Can you work these out from the model? Positions are in its coordinate system, mm. A direction names the side the tool comes from. Round coordinates to 2 decimals unless told otherwise and drop trailing zeros. Order: outer loops, then holes, each group sorted by start corner. A loop starts at its lowest first (then second) coordinate and runs counter-clockwise, first axis right, second up. Notation, with made-up numbers: M 86,74 L 106,74 A34 ccw 106,104 Z; hole C 21.5,-16.75 d3. An arc over 180 degrees is marked long. Answer as a JSON object with one key per item and string values. Group by question number.
```python
from build123d import *

# Parameters (mm, degrees)
ESQUISSE1_W                  = 62
ESQUISSE1_H                  = 62
BOSS_EXTRU_1_DEPTH           = 68
ESQUISSE2_R                  = 19
BOSS_EXTRU_2_DEPTH           = 4
ESQUISSE3_R                  = 8
BOSS_EXTRU_3_DEPTH           = 5
ENL_V_MAT_EXTRU_1_DEPTH      = 111.959452053
ENL_V_MAT_EXTRU_1_DEPTH_BACK = 111.959452053
ESQUISSE4_R                  = 3.6
CHANFREIN1_SIZE              = 3
ESQUISSE5_W                  = 20
ESQUISSE5_H                  = 9.5
BOSS_EXTRU_4_DEPTH           = 68
ESQUISSE6_R                  = 4.7625
ENL_V_MAT_EXTRU_2_DEPTH      = 5
ESQUISSE7_R                  = 5
ENL_V_MAT_EXTRU_3_DEPTH      = 70
CONG_1_R                     = 0.5


with BuildPart() as part:
    # Esquisse1 → Boss.-Extru.1 (new body)
    with BuildSketch(Plane.XY):
        with Locations((31, 31)):
            Rectangle(ESQUISSE1_W, ESQUISSE1_H)
    extrude(amount=BOSS_EXTRU_1_DEPTH)

    # Esquisse2 → Boss.-Extru.2 (add)
    with BuildSketch(Plane.XY.offset(68)):
        with Locations(Location((31, 31, 0), (0, 0, 180))):
            Circle(ESQUISSE2_R)
    extrude(amount=BOSS_EXTRU_2_DEPTH)

    # Esquisse3 → Boss.-Extru.3 (add)
    with BuildSketch(Plane.XY.offset(72)):
        with Locations((31, 31)):
            Circle(ESQUISSE3_R)
    extrude(amount=BOSS_EXTRU_3_DEPTH)

    # Esquisse4 → Enlèv. mat.-Extru.1 (cut, two sides: drawn at the far end of the back side and taken through both)
    with BuildSketch(Plane.XY.offset(68).offset(-ENL_V_MAT_EXTRU_1_DEPTH_BACK)):
        with Locations((7, 55)):
            Circle(ESQUISSE4_R)
        with Locations(Location((55, 55, 0), (0, 0, 180))):
            Circle(ESQUISSE4_R)
        with Locations((55, 7)):
            Circle(ESQUISSE4_R)
        with Locations(Location((7, 7, 0), (0, 0, 180))):
            Circle(ESQUISSE4_R)
    extrude(amount=ENL_V_MAT_EXTRU_1_DEPTH + ENL_V_MAT_EXTRU_1_DEPTH_BACK, mode=Mode.SUBTRACT)

    # Chanfrein1
    chanfrein1_edges = [part.edges().sort_by_distance(p)[0] for p in [
        (0, 62, 34),
        (62, 62, 34),
        (62, 0, 34),
        (0, 0, 34),
    ]]
    chamfer(chanfrein1_edges, length=CHANFREIN1_SIZE)

    # Esquisse5 → Boss.-Extru.4 (add)
    with BuildSketch(Plane.XY.offset(68)):
        with Locations((31, 66.75)):
            Rectangle(ESQUISSE5_W, ESQUISSE5_H)
    extrude(amount=-BOSS_EXTRU_4_DEPTH)

    # Esquisse6 → Enlèv. mat.-Extru.2 (cut)
    with BuildSketch(Plane(origin=(0, 71.5, 0), x_dir=(1, 0, 0), z_dir=(0, 1, 0))):
        with Locations(Location((31, -57.5, 0), (0, 0, 270))):
            Circle(ESQUISSE6_R)
        with Locations(Location((31, -10.5, 0), (0, 0, 90))):
            Circle(ESQUISSE6_R)
    extrude(amount=-ENL_V_MAT_EXTRU_2_DEPTH, mode=Mode.SUBTRACT)

    # Esquisse7 → Enlèv. mat.-Extru.3 (cut)
    with BuildSketch(Plane.XY.offset(77)):
        with Locations((31, 31)):
            Circle(ESQUISSE7_R)
    extrude(amount=-ENL_V_MAT_EXTRU_3_DEPTH, mode=Mode.SUBTRACT)

    # Congé1
    cong_1_edges = [part.edges().sort_by_distance(p)[0] for p in [
        (50, 31, 72),
    ]]
    fillet(cong_1_edges, radius=CONG_1_R)


solid = part.part
```
1) For pin 1 (14.5 mm diameter, centred on x = 53.5, z = 37, fed in from +Y); pin 2 (11.5 mm diameter, centred on x = 7, y = 7, fed in from +Z); pin 3 (8 mm diameter, centred on x = 32.5, y = 32.5, fed in from +Z); pin 4 (5 mm diameter, centred on y = 66, z = 40.5, fed in from -X), each with a flat end and sliding along its axis, tell me the tip position at first contact or that it passes through.
2) If we section it at D-D on y = 31: Write out the boundary of the cut face in (x, z).
3) If we section it at B-B on z = 28: Write out the boundary of the cut face in (x, y).
4) Which directions (+Z, -Z, +X, -X, +Y, -Y) give clear straight access to the entire face, cutting with the end or side of a thin tool? Please do faces 4 (the face through (16.8, 44.2, 68)), 5 (the face through (35.225, 69.035, 8.302)), 6 (the face through (21, 67, 34)).
5) I need wall thicknesses on line 1 along Y through (x, z) = (7, 43); line 2 along Y through (x, z) = (9.5, 46); line 3 along Y through (x, z) = (31, 12). Which ranges of each line are inside material? Lowest first, please.
6) We'd pull the mould along Y, two halves only. Please class faces 1 (the face through (53.065, 51.964, 33.524)), 2 (the face through (61, 60, 34)), 3 (the face through (61, 2, 34)): +Y half, -Y half, draft (parallel to the pull), parting line (faces both ways), or undercut.
7) If we section it at A-A on y = 55: Write out the boundary of the cut face in (x, z), plus the area to 3 significant figures.
Findings:
{
 "1": {"pin 1": "stops at y = 62", "pin 2": "stops at z = 68", "pin 3": "stops at z = 77", "pin 4": "stops at x = 21"},
 "2": {"outline": "M 0,0 L 62,0 L 62,68 L 50,68 L 50,71.5 A0.5 ccw 49.5,72 L 39,72 L 39,77 L 36,77 L 36,7 L 26,7 L 26,77 L 23,77 L 23,72 L 12.5,72 A0.5 ccw 12,71.5 L 12,68 L 0,68 Z"},
 "3": {"outline": "M 0,3 L 3,0 L 59,0 L 62,3 L 62,59 L 59,62 L 41,62 L 41,71.5 L 21,71.5 L 21,62 L 3,62 L 0,59 Z; hole C 7,7 d7.2; hole C 7,55 d7.2; hole C 31,31 d10; hole C 55,7 d7.2; hole C 55,55 d7.2"},
 "4": {"face 4": "+Z", "face 5": "+Y", "face 6": "+Z, -Z, -X, +Y"},
 "5": {"line 1": "y = 0 to 3.4, 10.6 to 51.4, 58.6 to 62", "line 2": "y = 0 to 4.41, 9.59 to 52.41, 57.59 to 62", "line 3": "y = 0 to 26, 36 to 66.5"},
 "6": {"face 1": "undercut", "face 2": "+Y half", "face 3": "-Y half"},
 "7": {"outline": "M 0,0 L 3.4,0 L 3.4,68 L 0,68 Z; M 10.6,0 L 51.4,0 L 51.4,68 L 10.6,68 Z; M 58.6,0 L 62,0 L 62,68 L 58.6,68 Z", "area": "3,240 mm^2"}
}
